The model under review builds one solid part; all positions refer to its coordinate system, in mm. Coordinates: 2 decimals unless noted, no trailing zeros. Write each loop counter-clockwise with the first axis right and the second up, starting at its lowest first coordinate (ties: lowest second). Pieces come first, ordered by that corner, then holes. Notation, with made-up numbers: M 4.5,16 L 32.5,16 A15 cw 32.5,25 Z; hole C -4,-25.75 d6. An arc over 180 degrees is marked long. Answer as a JSON object with one key per item and string values.
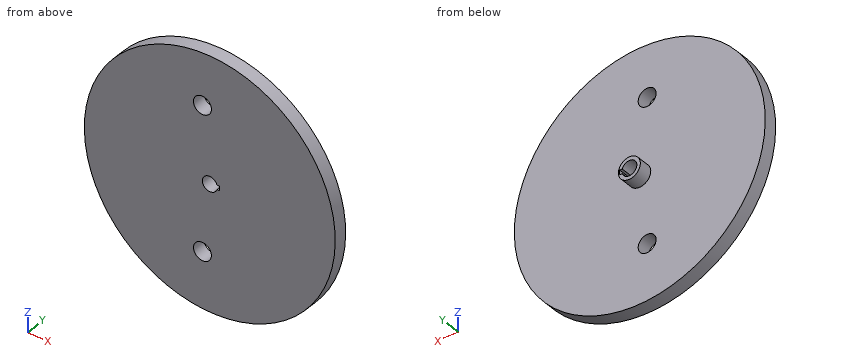
```python
from build123d import *

# Parameters (mm, degrees)
SKETCH1_R           = 140
BOSS_EXTRUDE1_DEPTH = 30.25
SKETCH2_R           = 36.5
SKETCH2_R_2         = 12.2445076
CUT_EXTRUDE1_DEPTH  = 15.125
SKETCH3_R           = 150
SKETCH3_R_2         = 12.938699975
CUT_EXTRUDE3_DEPTH  = 60
SKETCH4_R           = 10
CUT_EXTRUDE4_DEPTH  = 20


with BuildPart() as part:
    # Sketch1 → Boss-Extrude1 (new body)
    with BuildSketch(Plane(origin=(0, 0, 0), x_dir=(1, 0, 0), z_dir=(0, 1, 0))):
        with Locations(Location((0, 0, 0), (0, 0, 270))):
            Circle(SKETCH1_R)
        with BuildLine():
            Line((10.74, 0), (10.74, 2.5))
            Line((10.74, 2.5), (7.956481634, 2.5))
            ThreePointArc((7.956481634, 2.5), (-8.34, 0), (7.956481634, -2.5))
            Line((7.956481634, -2.5), (10.74, -2.5))
            Line((10.74, -2.5), (10.74, 0))
        make_face(mode=Mode.SUBTRACT)
    extrude(amount=BOSS_EXTRUDE1_DEPTH)

    # Sketch2 → Cut-Extrude1 (cut)
    with BuildSketch(Plane(origin=(0, 30.25, 0), x_dir=(1, 0, 0), z_dir=(0, 1, 0))):
        with Locations(Location((0, 0, 0), (0, 0, 270))):
            Circle(SKETCH2_R)
        with Locations(Location((0, 0, 0), (0, 0, 270))):
            Circle(SKETCH2_R_2, mode=Mode.SUBTRACT)
    extrude(amount=-CUT_EXTRUDE1_DEPTH, mode=Mode.SUBTRACT)

    # Sketch3 → Cut-Extrude3 (cut)
    with BuildSketch(Plane(origin=(0, 15.125, 0), x_dir=(1, 0, 0), z_dir=(0, 1, 0))):
        Circle(SKETCH3_R)
        Circle(SKETCH3_R_2, mode=Mode.SUBTRACT)
    extrude(amount=CUT_EXTRUDE3_DEPTH, mode=Mode.SUBTRACT)

    # Sketch4 → Cut-Extrude4 (cut)
    with BuildSketch(Plane(origin=(0, 0, 0), x_dir=(-1, 0, 0), z_dir=(0, -1, 0))):
        with Locations(Location((8.202870942, 77.402383207, 0), (0, 0, 90))):
            Circle(SKETCH4_R)
        with Locations(Location((8.202870942, -82.387978989, 0), (0, 0, 90))):
            Circle(SKETCH4_R)
    extrude(amount=-CUT_EXTRUDE4_DEPTH, mode=Mode.SUBTRACT)


solid = part.part
```
(1) Wall thickness on line 1 along X through (y, z) = (19, 0); line 2 along X through (y, z) = (6, 0); line 3 along Y through (x, z) = (-15, -103.5) (3 decimals): over which ranges is each line inside the solid? List them lowest first. Write a range as from..to.
Results list:
{"line 1": "-12.24..-8.34, 10.74..12.24", "line 2": "-140..-8.34, 10.74..140", "line 3": "0..15.125"}
(2) Add section A-A on z = 82. Give the boundary of the cut face in (x, y) (3 decimals).
Results list:
{"outline": "M -113.472,0 L -18.195,0 L -18.195,15.125 L -113.472,15.125 Z; M 1.79,0 L 113.472,0 L 113.472,15.125 L 1.79,15.125 Z"}
(3) For pin 1 Ø23 at (x, z) = (-8.2, 82.39) entering from +Y (3 decimals); pin 2 Ø3 at (x, y) = (83, 17) entering from +Z; pin 3 Ø1 at (y, z) = (15, 48) entering from +X; pin 4 Ø3 at (x, y) = (10, 13) entering from -Z, all flat-tipped, find the tip position at first contact; note any pin that passes through.
Results list:
{"pin 1": "y = 15.125", "pin 2": "through", "pin 3": "x = 131.7", "pin 4": "z = -139.74"}
(4) Add section D-D on z = -54.5. Give the boundary of the cut face in (x, y) (3 decimals).
Results list:
{"outline": "M -128.956,0 L 128.956,0 L 128.956,15.125 L -128.956,15.125 Z"}
(5) Add section C-C on x = 116.5. Give the boundary of the cut face in (y, z) (3 decimals).
Results list:
{"outline": "M 0,-77.639 L 15.125,-77.639 L 15.125,77.639 L 0,77.639 Z"}
(6) Add section B-B on y = 20. Give the boundary of the cut face in (x, z).
Results list:
{"outline": "C 0,0 d24.49; hole M 7.96,-2.5 L 10.74,-2.5 L 10.74,2.5 L 7.96,2.5 A8.34 ccw long Z"}
